Autodesk Inventor part; units mm, degrees
ref_plane "YZ Plane" through (0, 0, 0) normal (1, 0, 0) x (0, 1, 0)
ref_plane "XZ Plane" through (0, 0, 0) normal (0, 1, 0) x (-1, 0, 0)
ref_plane "XY Plane" through (0, 0, 0) normal (0, 0, 1) x (1, 0, 0)
sketch "Sketch1" plane through (0, 0, 0) normal (0, 1, 0) x (-1, 0, 0)
  line L0 (0, 0) -> (80, 0)
  line L1 (80, 0) -> (80, 200)
  line L2 (80, 200) -> (0, 200)
  line L3 (0, 200) -> (0, 0)
  dimension "d0" = 80
  dimension "d1" = 200
extrude "Extrusion1" add sketch "Sketch1" along normal blind 40
fillet "Fillet1" radius 10 8 edges at (0, 40, 100) (-40, 40, 200) (-80, 40, 100) (-40, 40, 0) (0, 20, 0) (0, 20, 200) (-80, 20, 200) (-80, 20, 0)
sketch "Sketch2" plane through (0, 40, 0) normal (0, 1, 0) x (1, 0, 0)
  line L0 (-68, -190) -> (-12, -190)
  line L1 (-10, -188) -> (-10, -12)
  line L2 (-12, -10) -> (-68, -10)
  line L3 (-70, -12) -> (-70, -188)
  line L4 (-70, -10) -> (-10, -10)
  line L5 (-10, -10) -> (-10, -190)
  arc A0 (-70, -188) -> (-68, -190) centre (-68, -188) ccw
  arc A1 (-68, -10) -> (-70, -12) centre (-68, -12) ccw
  arc A2 (-10, -12) -> (-12, -10) centre (-12, -12) ccw
  arc A3 (-12, -190) -> (-10, -188) centre (-12, -188) ccw
  point P0 (0, 0)
  point P1 (-70, -100)
  point P2 (-40, -10)
  dimension "d5" = 90
  dimension "d6" = 180
  dimension "d7" = 30
  dimension "d8" = 60
  dimension "d9" = 2
extrude "Extrusion2" cut sketch "Sketch2" against normal blind 6 contours A0 L3 A1 L2 A2 L1 A3 L0
properties part number "lcd screen"
Verification items for the finished model (mm, model axes). A direction names the side the tool comes from. Round coordinates to 2 decimals unless told otherwise and drop trailing zeros. Loops run counter-clockwise (first coordinate to the right, second up) from the corner with the lowest first, then second, coordinate; pieces in that order, holes last. Notation, with made-up numbers: (-28.75, -25) - (18.25, -25) arc R25 cw to (18.25, 9) - close; hole circle Ø2 at (58, -39.5). An arc over 180 degrees is marked (long way). Use a Markdown table: item, result. Add a question column.
1. Access from +Z, -Z, +X, -X, +Y, -Y to the whole of each face (thin tool, end or side, straight path). Record for faces 1 (the face through (-76.99, 37.15, 101.26)), 2 (the face through (-40, 37, 10)).
2. Thickness scan on probe 1 along Y at (x, z) = (-22.5, 99); probe 2 along X at (y, z) = (35, 54.5); probe 3 along X at (y, z) = (38.5, 136.5). Record the ranges inside material, lowest first. Write a range as [from, to].
3. Section check A-A, the plane z = 70. Record the boundary of the cut face in (x, y), plus the area to 3 significant figures.
4. Section check B-B, the plane x = -56.5. Record the boundary of the cut face in (y, z).
5. Release check for a two-part mould opening along X. For faces 3 (the face through (-39, 0, 101)), 4 (the face through (-70, 37, 99)), 5 (the face through (-80, 15, 99)) record: released by +X, released by -X, zero draft, split by the parting line, or undercut.
6. Gauge pin test, flat ends, axial feed: pin 1 (3 mm diameter, centred on x = -46, y = 36, fed in from -Z); pin 2 (12 mm diameter, centred on y = 30, z = 89, fed in from +X); pin 3 (5 mm diameter, centred on y = 36.5, z = 107.5, fed in from +X); pin 4 (3 mm diameter, centred on x = -21, z = 69, fed in from +Y). Record the tip position at first contact, or that the pin passes through.
Checks:
| question | item | result |
|---|---|---|
| 1 | face 1 | +Z, -Z, -X, +Y |
| 1 | face 2 | +Y |
| 2 | probe 1 | y = [0, 34] |
| 2 | probe 2 | x = [-78.66, -70], [-10, -1.34] |
| 2 | probe 3 | x = [-75.27, -70], [-10, -4.73] |
| 3 | outline | (-80, 0) - (0, 0) - (0, 30) arc R10 ccw to (-10, 40) - (-10, 34) - (-70, 34) - (-70, 40) arc R10 ccw to (-80, 30) - close |
| 3 | area | 2,800 mm^2 |
| 4 | outline | (0, 0) - (30, 0) arc R10 ccw to (40, 10) - (34, 10) - (34, 190) - (40, 190) arc R10 ccw to (30, 200) - (0, 200) - close |
| 5 | face 3 | zero draft |
| 5 | face 4 | undercut |
| 5 | face 5 | released by -X |
| 6 | pin 1 | stops at z = 1.07 |
| 6 | pin 2 | stops at x = 0 |
| 6 | pin 3 | stops at x = -0.83 |
| 6 | pin 4 | stops at y = 34 |
